Can you work these out from the model? Positions are in its coordinate system, mm. A direction names the side the tool comes from. Round coordinates to 2 decimals unless told otherwise and drop trailing zeros. Write each loop counter-clockwise with the first axis right and the second up, starting at its lowest first coordinate (ties: lowest second). Pieces come first, ordered by that corner, then holes.
Q1. I'm going to push flat-ended pins straight in: pin 1 Ø1 at (x, y) = (-8, -5) entering from -Z; pin 2 Ø2 at (x, y) = (0, -11) entering from +Z; pin 3 Ø0.6 at (y, z) = (-11, 16) entering from +X; pin 4 Ø1.5 at (x, z) = (26, 17.5) entering from -Y. Where does each tip first touch, or does it pass through?
Q2. If we section it at D-D (y = 0): Give the number of separate pieces and of enclosed holes in the cut face, plus the area to 3 significant figures.
Q3. If we section it at C-C (z = 6.75): Please give me the cut outline in (x, y), plus the area to 3 significant figures.
Q4. If we section it at A-A (z = 2.5): Please give me the cut outline in (x, y), plus the area to 3 significant figures.
Q5. We'd pull the mould along Z, two halves only. Please class faces 1 (the cylindrical face through (-25.9, -10.5, 6.9)), 2 (the flat face through (-15, -11, 17)), 3 (the cylindrical face through (27.715, 0.077, -1.699)), 4 (the flat face through (-25.5, 0, 16)): +Z half, -Z half, draft (parallel to the pull), parting line (faces both ways), or undercut.
Q6. For faces 5 (the cylindrical face through (3.7, -2.93, 1.97)), 6 (the flat face through (-17, -12, 16)), 7 (the flat face through (27, -5, 17)), 8 (the flat face through (25.5, 0, 16)), 9 (the flat face through (12, -12, 16)), which set-ups out of +Z, -Z, +X, -X, +Y, -Y let a thin tool reach every point of the face, with its end or its side?
Q7. Please list where these lines run through material, in increasing order: line 1 along Y through (x, z) = (13, 0.3); line 2 along Y through (x, z) = (10.5, 0.5); line 3 along Y through (x, z) = (-19, 11.5).
Q8. If we section it at B-B (x = 13): Please give me the cut outline in (y, z).
from build123d import *

# Parameters (mm, degrees)
SKETCH2_W                      = 56
SKETCH2_H                      = 25
SKETCH2_W_2                    = 46
SKETCH2_H_2                    = 21
BOX_DEPTH                      = 15
SKETCH3_W                      = 56
SKETCH3_H                      = 25
FRONT_DEPTH                    = 2
SKETCH8_R                      = 9.75
BOSS_EXTRUDE7_DEPTH            = 4
SKETCH1_R                      = 8.25
CUT_EXTRUDE1_DEPTH             = 35.135758377
CUT_EXTRUDE1_DIRECTION_2_REACH = 36.136
FILLET1_R                      = 7
BOSS_EXTRUDE3_DEPTH            = 11
FILLET2_R                      = 1
FILLET3_R                      = 1
SKETCH5_W                      = 2.5
SKETCH5_H                      = 10
BOSS_EXTRUDE4_DEPTH            = 4
SKETCH6_W                      = 5
SKETCH6_H                      = 2
BOSS_EXTRUDE5_DEPTH            = 2
BOSS_EXTRUDE6_DEPTH            = 10


with BuildPart() as part:
    # Sketch2 → Box (new body)
    with BuildSketch(Plane.XY):
        Rectangle(SKETCH2_W, SKETCH2_H)
        Rectangle(SKETCH2_W_2, SKETCH2_H_2, mode=Mode.SUBTRACT)
    extrude(amount=BOX_DEPTH)

    # Sketch3 → Front (add)
    with BuildSketch(Plane(origin=(0, 0, 0), x_dir=(-1, 0, 0), z_dir=(0, 0, -1))):
        Rectangle(SKETCH3_W, SKETCH3_H)
    extrude(amount=FRONT_DEPTH)

    # Sketch8 → Boss-Extrude7 (add)
    with BuildSketch(Plane.XY):
        with Locations(Location((-13, 0, 0), (0, 0, 180))):
            Circle(SKETCH8_R)
        with Locations(Location((13, 0, 0), (0, 0, 180))):
            Circle(SKETCH8_R)
    extrude(amount=BOSS_EXTRUDE7_DEPTH)

    # Sketch1 → Cut-Extrude1 (cut)
    with BuildSketch(Plane.XY):
        with Locations(Location((-13, 0, 0), (0, 0, 180))):
            Circle(SKETCH1_R)
        with Locations(Location((13, 0, 0), (0, 0, 180))):
            Circle(SKETCH1_R)
    extrude(amount=-CUT_EXTRUDE1_DEPTH, mode=Mode.SUBTRACT)

    # Sketch1 → Cut-Extrude1 direction 2 (cut, up to next)
    with BuildSketch(Plane.XY, mode=Mode.PRIVATE) as cut_extrude1_direction_2_sk1:
        with Locations(Location((-13, 0, 0), (0, 0, 180))):
            Circle(SKETCH1_R)
    cut_extrude1_direction_2_tool1 = extrude(cut_extrude1_direction_2_sk1.sketch, amount=CUT_EXTRUDE1_DIRECTION_2_REACH, mode=Mode.PRIVATE) & part.part
    # Sketch1 → Cut-Extrude1 direction 2 (cut, up to next)
    with BuildSketch(Plane.XY, mode=Mode.PRIVATE) as cut_extrude1_direction_2_sk2:
        with Locations(Location((13, 0, 0), (0, 0, 180))):
            Circle(SKETCH1_R)
    cut_extrude1_direction_2_tool2 = extrude(cut_extrude1_direction_2_sk2.sketch, amount=CUT_EXTRUDE1_DIRECTION_2_REACH, mode=Mode.PRIVATE) & part.part
    add(cut_extrude1_direction_2_tool1.solids().sort_by_distance((-13, 0, 0))[0], mode=Mode.SUBTRACT)
    add(cut_extrude1_direction_2_tool2.solids().sort_by_distance((13, 0, 0))[0], mode=Mode.SUBTRACT)

    # Fillet1
    fillet1_edges = [part.edges().sort_by_distance(p)[0] for p in [
        (-28, 12.5, 6.5),
        (28, 12.5, 6.5),
        (28, -12.5, 6.5),
        (-28, -12.5, 6.5),
    ]]
    fillet(fillet1_edges, radius=FILLET1_R)

    # Sketch4 → Boss-Extrude3 (add)
    with BuildSketch(Plane.XY):
        with BuildLine():
            Line((-23, 6.5), (-23, 10.5))
            Line((-23, 10.5), (-19, 10.5))
            ThreePointArc((-19, 10.5), (-20.171572875, 7.671572875), (-23, 6.5))
        make_face()
        with BuildLine():
            Line((19, 10.5), (23, 10.5))
            Line((23, 10.5), (23, 6.5))
            ThreePointArc((23, 6.5), (20.171572875, 7.671572875), (19, 10.5))
        make_face()
        with BuildLine():
            Line((-23, -6.5), (-23, -10.5))
            Line((-23, -10.5), (-19, -10.5))
            ThreePointArc((-19, -10.5), (-20.171572875, -7.671572875), (-23, -6.5))
        make_face()
        with BuildLine():
            Line((23, -6.5), (23, -10.5))
            Line((23, -10.5), (19, -10.5))
            ThreePointArc((19, -10.5), (20.171572875, -7.671572875), (23, -6.5))
        make_face()
    extrude(amount=BOSS_EXTRUDE3_DEPTH)

    # Fillet2
    fillet2_edges = [part.edges().sort_by_distance(p)[0] for p in [
        (0, 12.5, -2),
        (28, 0, -2),
        (0, -12.5, -2),
        (-28, 0, -2),
        (-25.949747468, -10.449747468, -2),
        (25.949747468, -10.449747468, -2),
        (-25.949747468, 10.449747468, -2),
        (25.949747468, 10.449747468, -2),
    ]]
    fillet(fillet2_edges, radius=FILLET2_R)

    # Fillet3
    fillet3_edges = [part.edges().sort_by_distance(p)[0] for p in [
        (-4.75, 0, -2),
        (21.25, 0, -2),
    ]]
    fillet(fillet3_edges, radius=FILLET3_R)

    # Sketch5 → Boss-Extrude4 (add)
    with BuildSketch(Plane.XY.offset(15)):
        with Locations((-26.75, 0)):
            Rectangle(SKETCH5_W, SKETCH5_H)
        with Locations((26.75, 0)):
            Rectangle(SKETCH5_W, SKETCH5_H)
    extrude(amount=BOSS_EXTRUDE4_DEPTH)

    # Sketch6 → Boss-Extrude5 (add)
    with BuildSketch(Plane.XY.offset(15)):
        with Locations((-14.5, -11.5)):
            Rectangle(SKETCH6_W, SKETCH6_H)
        with Locations((14.5, -11.5)):
            Rectangle(SKETCH6_W, SKETCH6_H)
    extrude(amount=BOSS_EXTRUDE5_DEPTH)

    # Sketch7 → Boss-Extrude6 (add)
    with BuildSketch(Plane(origin=(0, 5, 0), x_dir=(1, 0, 0), z_dir=(0, 1, 0))):
        Polygon((-25.5, -17), (-25, -19), (-25.5, -19), align=None)
        Polygon((25.5, -19), (25.5, -17), (25, -19), align=None)
    extrude(amount=-BOSS_EXTRUDE6_DEPTH)


solid = part.part
A:
1. pin 1: passes through
1. pin 2: stops at z = 15
1. pin 3: stops at x = 17
1. pin 4: stops at y = -5
2. separate pieces: 3
2. enclosed holes: 0
2. area: 240 mm2
3. outline: (-28, -5.5) arc R7 ccw to (-21, -12.5) - (21, -12.5) arc R7 ccw to (28, -5.5) - (28, 5.5) arc R7 ccw to (21, 12.5) - (-21, 12.5) arc R7 ccw to (-28, 5.5) - close; hole (-23, -6.5) arc R4 cw to (-19, -10.5) - (19, -10.5) arc R4 cw to (23, -6.5) - (23, 6.5) arc R4 cw to (19, 10.5) - (-19, 10.5) arc R4 cw to (-23, 6.5) - close
3. area: 442 mm2
4. outline: (-28, -5.5) arc R7 ccw to (-21, -12.5) - (21, -12.5) arc R7 ccw to (28, -5.5) - (28, 5.5) arc R7 ccw to (21, 12.5) - (-21, 12.5) arc R7 ccw to (-28, 5.5) - close; circle Ø19.5 at (-13, 0); circle Ø19.5 at (13, 0); hole (-23, -6.5) arc R4 cw to (-19, -10.5) - (19, -10.5) arc R4 cw to (23, -6.5) - (23, 6.5) arc R4 cw to (19, 10.5) - (-19, 10.5) arc R4 cw to (-23, 6.5) - close; hole circle Ø16.5 at (-13, 0); hole circle Ø16.5 at (13, 0)
4. area: 612 mm2
5. face 1: draft
5. face 2: +Z half
5. face 3: -Z half
5. face 4: undercut
6. face 5: +Z
6. face 6: +Z, -X, +Y, -Y
6. face 7: +Z, +X, -X, -Y
6. face 8: +Y, -Y
6. face 9: +Z, +Y, -Y
7. line 1: y = -12.5 to -10.5, -9.75 to -8.25, 8.25 to 9.75, 10.5 to 12.5
7. line 2: y = -12.5 to -10.5, -9.42 to -7.86, 7.86 to 9.42, 10.5 to 12.5
7. line 3: y = -12.5 to -10.5, 10.5 to 12.5
8. outline: (-12.5, -1) arc R1 ccw to (-11.5, -2) - (-9.25, -2) arc R1 ccw to (-8.25, -1) - (-8.25, 4) - (-9.75, 4) - (-9.75, 0) - (-10.5, 0) - (-10.5, 17) - (-12.5, 17) - close; (8.25, -1) arc R1 ccw to (9.25, -2) - (11.5, -2) arc R1 ccw to (12.5, -1) - (12.5, 15) - (10.5, 15) - (10.5, 0) - (9.75, 0) - (9.75, 4) - (8.25, 4) - close
